from build123d import *

# Parameters (mm, degrees)
F0_W            = 43.0059846
F0_H            = 43.0059846
F0_R            = 1.5
F0_R_2          = 11.2530001
F1_DEPTH        = 2.79375108
F2_SIZE         = 6.0030106
F4_DEPTH        = 2.79375108
F4_COPIES_COUNT = 4


# Not quite as in the source:
# - a pattern or mirror of a feature is missing from the dataset's text; its kind, count and spacing are read off the source's solid


with BuildPart() as f1:
    # F0 (on Top) → F1 (new body)
    with BuildSketch(Plane.XY):
        with Locations((21.5029923, 21.5029923)):
            Rectangle(F0_W, F0_H)
        with Locations((6.0029979, 6.0029979)):
            Circle(F0_R, mode=Mode.SUBTRACT)
        with Locations((21.5029923, 21.5029923)):
            Circle(F0_R_2, mode=Mode.SUBTRACT)
        with Locations((37.0029867, 6.0029979)):
            Circle(F0_R, mode=Mode.SUBTRACT)
        with Locations((6.0029979, 37.0029867)):
            Circle(F0_R, mode=Mode.SUBTRACT)
        with Locations((37.0029867, 37.0029867)):
            Circle(F0_R, mode=Mode.SUBTRACT)
    extrude(amount=F1_DEPTH)

    # F2
    f2_edges = [f1.edges().sort_by_distance(p)[0] for p in [
        (0, 0, 1.396876),
        (0, 43.005985, 1.396876),
        (43.005985, 0, 1.396876),
        (43.005985, 43.005985, 1.396876),
    ]]
    chamfer(f2_edges, length=F2_SIZE)

    # F3 (on face) → F4 (cut, through all)
    with BuildSketch(Plane.XY.offset(2.79375108)):
        with BuildLine():
            ThreePointArc((7.2356236023, 32.4027649523), (5.1176370603, 32.3235056996), (3.175, 33.171037571))
            Line((3.175, 33.171037571), (3.175, 9.834947029))
            ThreePointArc((3.175, 9.834947029), (5.1176370603, 10.6824789004), (7.2356236023, 10.6032196477))
            Line((7.2356236023, 10.6032196477), (9.7569670059, 13.1245630513))
            ThreePointArc((9.7569670059, 13.1245630513), (7.0749922, 21.5029923), (9.7569670059, 29.8814215487))
            Line((9.7569670059, 29.8814215487), (7.2356236023, 32.4027649523))
        make_face()
    f4 = extrude(amount=-F4_DEPTH, mode=Mode.SUBTRACT)

    # F4_copies: F4 ×4 about axis
    f4_copies_axis = Axis((21.502992, 21.502992, 0), (0, 0, 1))
    for i in range(1, F4_COPIES_COUNT):
        add(f4.rotate(f4_copies_axis, i * 360 / F4_COPIES_COUNT), mode=Mode.SUBTRACT)


solid = f1.part
Part model, mm, in its own coordinate system. A direction names the side the tool comes from. Coordinates: 2 decimals unless noted, no trailing zeros. Loops run counter-clockwise (first coordinate to the right, second up) from the corner with the lowest first, then second, coordinate; pieces in that order, holes last. Notation, with made-up numbers: M 9.5,30 L 55.5,30 A26 cw 55.5,44 Z; hole C 40,-22 d7. An arc over 180 degrees is marked long. Use a Markdown table: item, result. Add a question column.
Q1. Probe L1, parallel to Y at x = 15, z = 1 (3 decimals); L2, parallel to X at y = 38, z = 0.35; L3, parallel to X at y = 11.5, z = 0.95 (3 decimals). List the from-to ranges inside material, lowest first.
Q2. Cut at C-C (x = 8). Write the cut outline in (y, z).
Q3. Cut at D-D (z = 1.8). Give the number of separate pieces and of enclosed holes in the cut face, and give its area (3 significant figures).
Q4. Mould opens along X. For faces 3 (the flat face through (21, 3.175, 1)), 4 (the flat face through (40.047, 3.044, 1.377)), 5 (the flat face through (21, 43.006, 1)) say: +X half, -X half, draft (parallel to the pull), parting line (faces both ways), or undercut.
Q5. Which spindle directions (+Z, -Z, +X, -X, +Y, -Y) get a long thin tool onto all of the face, cutting with end or side? Do faces 1 (the flat face through (43.006, 21, 1)), 2 (the flat face through (11.88, 8.51, 1.42)). Say none if no direction does.
Q6. Cut at A-A (x = 26). Write the cut outline in (y, z) (3 decimals).
Q7. Pin check, flat tip, straight feed: P1, Ø4, axis at x = 7, y = 29, coming from the +Z side. Stop position of the tip, or through.
Q8. Cut at B-B (y = 18). Write the cut outline in (x, z) (3 decimals).
Worked out:
| question | item | result |
|---|---|---|
| 1 | L1 | y = 0 to 3.175, 8.624 to 12.319, 30.687 to 34.382, 39.831 to 43.006 |
| 1 | L2 | x = 1 to 4.88, 7.12 to 10.66, 32.35 to 35.88, 38.12 to 42.01 |
| 1 | L3 | x = 0 to 3.175, 8.132 to 16.348, 26.658 to 34.874, 39.831 to 43.006 |
| 2 | outline | M 0,0 L 11.37,0 L 11.37,2.79 L 0,2.79 Z; M 16.42,0 L 26.59,0 L 26.59,2.79 L 16.42,2.79 Z; M 31.64,0 L 43.01,0 L 43.01,2.79 L 31.64,2.79 Z |
| 3 | separate pieces | 1 |
| 3 | enclosed holes | 9 |
| 3 | area | 923 mm2 |
| 4 | face 3 | undercut |
| 4 | face 4 | +X half |
| 4 | face 5 | draft |
| 5 | face 1 | +Z, -Z, +X, +Y, -Y |
| 5 | face 2 | +Z, -Z |
| 6 | outline | M 0,0 L 3.175,0 L 3.175,2.794 L 0,2.794 Z; M 7.794,0 L 11.188,0 L 11.188,2.794 L 7.794,2.794 Z; M 31.818,0 L 35.212,0 L 35.212,2.794 L 31.818,2.794 Z; M 39.831,0 L 43.006,0 L 43.006,2.794 L 39.831,2.794 Z |
| 7 | P1 | stops at z = 2.79 |
| 8 | outline | M 0,0 L 3.175,0 L 3.175,2.794 L 0,2.794 Z; M 7.507,0 L 10.809,0 L 10.809,2.794 L 7.507,2.794 Z; M 32.197,0 L 35.499,0 L 35.499,2.794 L 32.197,2.794 Z; M 39.831,0 L 43.006,0 L 43.006,2.794 L 39.831,2.794 Z |
